from build123d import *

# Parameters (mm, degrees)
SKETCH1_R           = 75
BOSS_EXTRUDE1_DEPTH = 5
BOSS_EXTRUDE2_DEPTH = 5
BOSS_EXTRUDE3_START = -5
BOSS_EXTRUDE3_DEPTH = 5
SKETCH6_R           = 1.5
CUT_EXTRUDE1_DEPTH  = 5
SKETCH7_R           = 2.9
CUT_EXTRUDE2_DEPTH  = 2.5
SKETCH8_R           = 0.6
CUT_EXTRUDE3_DEPTH  = 5
CIRPATTERN1_COUNT   = 4
SKETCH10_R          = 1.7
CUT_EXTRUDE4_DEPTH  = 3
CIRPATTERN2_COUNT   = 4
SKETCH11_R          = 2.5
CUT_EXTRUDE5_DEPTH  = 5
SKETCH12_R          = 1.4
CUT_EXTRUDE6_DEPTH  = 5
CIRPATTERN3_COUNT   = 4
SKETCH16_R          = 10.5
CUT_EXTRUDE10_DEPTH = 2.5
CUT_EXTRUDE11_DEPTH = 5
FILLET1_R           = 5
SKETCH19_R          = 15.25
CUT_EXTRUDE12_DEPTH = 2
SKETCH20_W          = 5
SKETCH20_H          = 4
CUT_EXTRUDE13_DEPTH = 2.5
SKETCH21_R          = 6.5
CUT_EXTRUDE14_DEPTH = 1.75


with BuildPart() as part:
    # Sketch1 → Boss-Extrude1 (new body)
    with BuildSketch(Plane(origin=(0, 0, 0), x_dir=(1, 0, 0), z_dir=(0, 1, 0))):
        with Locations(Location((0, 0, 0), (0, 0, 270))):
            Circle(SKETCH1_R)
    extrude(amount=BOSS_EXTRUDE1_DEPTH)

    # Sketch4 → Boss-Extrude2 (add)
    with BuildSketch(Plane.ZY.offset(25)):
        with BuildLine():
            Line((-13.582225242, 61.365780194), (-40, 5))
            Line((-40, 5), (40, 5))
            Line((40, 5), (13.582225242, 61.365780194))
            ThreePointArc((13.582225242, 61.365780194), (0, 70), (-13.582225242, 61.365780194))
        make_face()
    extrude(amount=BOSS_EXTRUDE2_DEPTH)

    # Sketch5 → Boss-Extrude3 (add)
    with BuildSketch(Plane.ZY.offset(-25).offset(BOSS_EXTRUDE3_START)):
        with BuildLine():
            Line((13.582225242, 61.365780194), (40, 5))
            Line((40, 5), (-40, 5))
            Line((-40, 5), (-13.582225242, 61.365780194))
            ThreePointArc((-13.582225242, 61.365780194), (0, 70), (13.582225242, 61.365780194))
        make_face()
    extrude(amount=BOSS_EXTRUDE3_DEPTH)

    # Sketch6 → Cut-Extrude1 (cut)
    with BuildSketch(Plane.ZY.offset(30)):
        with Locations((0, 55)):
            Circle(SKETCH6_R)
    extrude(amount=-CUT_EXTRUDE1_DEPTH, mode=Mode.SUBTRACT)

    # Sketch7 → Cut-Extrude2 (cut)
    with BuildSketch(Plane.ZY.offset(30)):
        with Locations((0, 55)):
            Circle(SKETCH7_R)
    extrude(amount=-CUT_EXTRUDE2_DEPTH, mode=Mode.SUBTRACT)

    # Sketch8 → Cut-Extrude3 (cut)
    with BuildSketch(Plane.ZY.offset(30)):
        with Locations((0, 62.25)):
            Circle(SKETCH8_R)
    cut_extrude3 = extrude(amount=-CUT_EXTRUDE3_DEPTH, mode=Mode.SUBTRACT)

    # CirPattern1: Cut-Extrude3 ×4 about axis
    cirpattern1_axis = Axis((0, 55, 0), (1, 0, 0))
    for i in range(1, CIRPATTERN1_COUNT):
        add(cut_extrude3.rotate(cirpattern1_axis, i * 360 / CIRPATTERN1_COUNT), mode=Mode.SUBTRACT)

    # Sketch10 → Cut-Extrude4 (cut)
    with BuildSketch(Plane.ZY.offset(30)):
        with Locations((0, 62)):
            Circle(SKETCH10_R)
    cut_extrude4 = extrude(amount=-CUT_EXTRUDE4_DEPTH, mode=Mode.SUBTRACT)

    # CirPattern2: Cut-Extrude4 ×4 about axis
    cirpattern2_axis = Axis((0, 55, 0), (1, 0, 0))
    for i in range(1, CIRPATTERN2_COUNT):
        add(cut_extrude4.rotate(cirpattern2_axis, i * 360 / CIRPATTERN2_COUNT), mode=Mode.SUBTRACT)

    # Sketch11 → Cut-Extrude5 (cut)
    with BuildSketch(Plane(origin=(0, 5, 0), x_dir=(1, 0, 0), z_dir=(0, 1, 0))):
        with Locations(Location((0, 0, 0), (0, 0, 270))):
            Circle(SKETCH11_R)
    extrude(amount=-CUT_EXTRUDE5_DEPTH, mode=Mode.SUBTRACT)

    # Sketch12 → Cut-Extrude6 (cut)
    with BuildSketch(Plane(origin=(0, 5, 0), x_dir=(1, 0, 0), z_dir=(0, 1, 0))):
        with Locations(Location((0, 12, 0), (0, 0, 270))):
            Circle(SKETCH12_R)
    cut_extrude6 = extrude(amount=-CUT_EXTRUDE6_DEPTH, mode=Mode.SUBTRACT)

    # CirPattern3: Cut-Extrude6 ×4 about axis
    cirpattern3_axis = Axis((0, 0, 0), (0, 1, 0))
    for i in range(1, CIRPATTERN3_COUNT):
        add(cut_extrude6.rotate(cirpattern3_axis, i * 360 / CIRPATTERN3_COUNT), mode=Mode.SUBTRACT)

    # Sketch16 → Cut-Extrude10 (cut)
    with BuildSketch(Plane(origin=(-25, 0, 0), x_dir=(0, 0, -1), z_dir=(1, 0, 0))):
        with Locations((0, 55)):
            Circle(SKETCH16_R)
    extrude(amount=-CUT_EXTRUDE10_DEPTH, mode=Mode.SUBTRACT)

    # Sketch18 → Cut-Extrude11 (cut)
    with BuildSketch(Plane(origin=(30, 0, 0), x_dir=(0, 0, -1), z_dir=(1, 0, 0))):
        with BuildLine():
            Line((-2.9, 55), (-2.9, 69.716996976))
            ThreePointArc((-2.9, 69.716996976), (0, 70), (2.9, 69.716996976))
            Line((2.9, 69.716996976), (2.9, 55))
            ThreePointArc((2.9, 55), (0, 52.1), (-2.9, 55))
        make_face()
    extrude(amount=-CUT_EXTRUDE11_DEPTH, mode=Mode.SUBTRACT)

    # Fillet1
    fillet1_edges = [part.edges().sort_by_distance(p)[0] for p in [
        (30, 5, 0),
        (27.5, 5, 40),
        (27.5, 5, -40),
        (25, 5, 0),
        (-25, 5, 0),
        (-27.5, 5, -40),
        (-27.5, 5, 40),
        (-30, 5, 0),
    ]]
    fillet(fillet1_edges, radius=FILLET1_R)

    # Sketch19 → Cut-Extrude12 (cut)
    with BuildSketch(Plane(origin=(0, 0, 0), x_dir=(-1, 0, 0), z_dir=(0, -1, 0))):
        with Locations(Location((0, 0, 0), (0, 0, 90))):
            Circle(SKETCH19_R)
    extrude(amount=-CUT_EXTRUDE12_DEPTH, mode=Mode.SUBTRACT)

    # Sketch20 → Cut-Extrude13 (cut)
    with BuildSketch(Plane(origin=(-25, 0, 0), x_dir=(0, 0, -1), z_dir=(1, 0, 0))):
        with Locations((0, 44.5)):
            Rectangle(SKETCH20_W, SKETCH20_H)
    extrude(amount=-CUT_EXTRUDE13_DEPTH, mode=Mode.SUBTRACT)

    # Sketch21 → Cut-Extrude14 (cut)
    with BuildSketch(Plane(origin=(0, 2, 0), x_dir=(-1, 0, 0), z_dir=(0, -1, 0))):
        with Locations(Location((0, 0, 0), (0, 0, 90))):
            Circle(SKETCH21_R)
    extrude(amount=-CUT_EXTRUDE14_DEPTH, mode=Mode.SUBTRACT)


solid = part.part
Source: CAD feature listing. Evaluate the final solid. Frame: model axes, mm. A direction names the side the tool comes from. Give positions to 0.01 mm unless a question says otherwise; leave off trailing zeros. Write each loop counter-clockwise with the first axis right and the second up, starting at its lowest first coordinate (ties: lowest second). Pieces come first, ordered by that corner, then holes. Notation, with made-up numbers: (-26, 1.5) -> (29, 1.5) arc R23 ccw to (29, 29.5) -> close; hole circle Ø6 at (50.5, -6.5). An arc over 180 degrees is marked (long way). Return JSON: item names as keys, results as strings. Group by question number.
1. Section D-D, the plane x = -59.5. Output: boundary loops of the cut face in (y, z).
2. Section B-B, the plane z = 25. Output: boundary loops of the cut face in (x, y).
3. Material intervals for line 1 (Y direction, x = 51.5, z = -52.5); line 2 (Y direction, x = -12, z = 6); line 3 (Z direction, x = -12, y = 3), sorted ascending. Write a range as from..to.
4. Pin query (flat end, axial travel): pin 1 Ø11.5 at (x, z) = (0, 0) entering from -Y; pin 2 Ø1.2 at (x, y) = (-26, 44) entering from -Z; pin 3 Ø10.5 at (y, z) = (59.5, -2) entering from +X; pin 4 Ø2 at (x, z) = (12, 0) entering from +Y. Return the tip coordinate at first contact, or that it passes through.
5. Section C-C, the plane y = 38. Output: boundary loops of the cut face in (x, z).
6. Access query for faces 1 (the face through (28, 62, 2.9)), 2 (the face through (-14.887, 0.986, 3.306)), 3 (the face through (-25, 27, -1)), 4 (the face through (-28.77, 53.3, -7.07)). Directions: +Z, -Z, +X, -X, +Y, -Y. A direction counts if a zero-diameter tool reaches every point of the face in a straight line with its end or side. Return the directions, or none.
7. Section A-A, the plane y = 26. Output: boundary loops of the cut face in (x, z), then the cut area to 3 significant figures.
8. Mould query, pull axis Z, two halves, no side actions, for faces 5 (the face through (-7, 2, 0)), 6 (the face through (28, 67, -9)), 7 (the face through (-23, 6, 1)). Classes: +Z half, -Z half, draft (parallel to the pull), parting line (faces both ways), or undercut.
Determined:
{
 "1": {"outline": "(0, -45.66) -> (5, -45.66) -> (5, 45.66) -> (0, 45.66) -> close"},
 "2": {"outline": "(-70.71, 0) -> (70.71, 0) -> (70.71, 5) -> (35, 5) arc R5 cw to (30, 10) -> (30, 37) -> (25, 37) -> (25, 10) arc R5 cw to (20, 5) -> (-20, 5) arc R5 cw to (-25, 10) -> (-25, 37) -> (-30, 37) -> (-30, 10) arc R5 cw to (-35, 5) -> (-70.71, 5) -> close"},
 "3": {"line 1": "y = 0..5", "line 2": "y = 2..5", "line 3": "z = -74.03..-1.4, 1.4..74.03"},
 "4": {"pin 1": "stops at y = 3.75", "pin 2": "stops at z = -22", "pin 3": "stops at x = 30", "pin 4": "passes through"},
 "5": {"outline": "(-30, -24.53) -> (-25, -24.53) -> (-25, 24.53) -> (-30, 24.53) -> close; (25, -24.53) -> (30, -24.53) -> (30, 24.53) -> (25, 24.53) -> close"},
 "6": {"face 1": "+X, +Y", "face 2": "-Y", "face 3": "+Z, -Z, +Y", "face 4": "-X"},
 "7": {"outline": "(-30, -30.16) -> (-25, -30.16) -> (-25, 30.16) -> (-30, 30.16) -> close; (25, -30.16) -> (30, -30.16) -> (30, 30.16) -> (25, 30.16) -> close", "area": "603 mm2"},
 "8": {"face 5": "undercut", "face 6": "-Z half", "face 7": "draft"}
}
